```python
from build123d import *

# Parameters (mm, degrees)
CYLINDER005_R     = 2
CYLINDER005_DEPTH = 10
CYLINDER004_R     = 2
CYLINDER004_DEPTH = 10
CYLINDER003_R     = 2
CYLINDER003_DEPTH = 10
CYLINDER002_R     = 2
CYLINDER002_DEPTH = 10
CYLINDER001_R     = 2
CYLINDER001_DEPTH = 10
CYLINDER_R        = 2
CYLINDER_DEPTH    = 10
BOX_W             = 20
BOX_H             = 14
BOX_DEPTH         = 10


with BuildPart() as cilindro005:
    # Cylinder005 → Cylinder005 (new body)
    with BuildSketch(Plane(origin=(16, 10, 0), x_dir=(1, 0, 0), z_dir=(0, 0, 1))):
        Circle(CYLINDER005_R)
    extrude(amount=CYLINDER005_DEPTH)


with BuildPart() as cilindro004:
    # Cylinder004 → Cylinder004 (new body)
    with BuildSketch(Plane(origin=(16, 4, 0), x_dir=(1, 0, 0), z_dir=(0, 0, 1))):
        Circle(CYLINDER004_R)
    extrude(amount=CYLINDER004_DEPTH)


with BuildPart() as cilindro003:
    # Cylinder003 → Cylinder003 (new body)
    with BuildSketch(Plane(origin=(10, 10, 0), x_dir=(1, 0, 0), z_dir=(0, 0, 1))):
        Circle(CYLINDER003_R)
    extrude(amount=CYLINDER003_DEPTH)


with BuildPart() as cilindro002:
    # Cylinder002 → Cylinder002 (new body)
    with BuildSketch(Plane(origin=(10, 4, 0), x_dir=(1, 0, 0), z_dir=(0, 0, 1))):
        Circle(CYLINDER002_R)
    extrude(amount=CYLINDER002_DEPTH)


with BuildPart() as cilindro001:
    # Cylinder001 → Cylinder001 (new body)
    with BuildSketch(Plane(origin=(4, 10, 0), x_dir=(1, 0, 0), z_dir=(0, 0, 1))):
        Circle(CYLINDER001_R)
    extrude(amount=CYLINDER001_DEPTH)


with BuildPart() as cilindro:
    # Cylinder → Cylinder (new body)
    with BuildSketch(Plane(origin=(4, 4, 0), x_dir=(1, 0, 0), z_dir=(0, 0, 1))):
        Circle(CYLINDER_R)
    extrude(amount=CYLINDER_DEPTH)


with BuildPart() as cut005:
    # Box → Box (new body)
    with BuildSketch(Plane.XY):
        with Locations((10, 7)):
            Rectangle(BOX_W, BOX_H)
    extrude(amount=BOX_DEPTH)

    # Cut: cut Cilindro
    add(cilindro.part, mode=Mode.SUBTRACT)

    # Cut001: cut Cilindro001
    add(cilindro001.part, mode=Mode.SUBTRACT)

    # Cut002: cut Cilindro002
    add(cilindro002.part, mode=Mode.SUBTRACT)

    # Cut003: cut Cilindro003
    add(cilindro003.part, mode=Mode.SUBTRACT)

    # Cut004: cut Cilindro004
    add(cilindro004.part, mode=Mode.SUBTRACT)

    # Cut005: cut Cilindro005
    add(cilindro005.part, mode=Mode.SUBTRACT)


solid = cut005.part
```
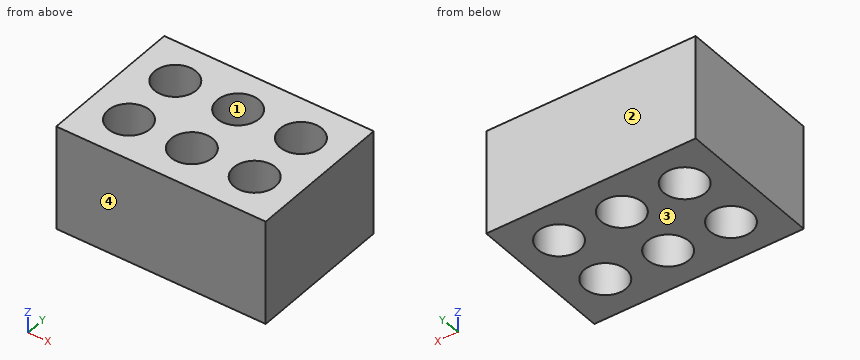
Geometry: final body of the model. Coordinates: model frame, mm. Face numbers are marked on the shaded views. Coordinates: 2 decimals unless noted, no trailing zeros. Loops run counter-clockwise (first coordinate to the right, second up) from the corner with the lowest first, then second, coordinate; pieces in that order, holes last. Notation, with made-up numbers: M 61,59.5 L 108,59.5 A12 cw 108,74.5 Z; hole C -28.75,-37.75 d8. An arc over 180 degrees is marked long. Put each result on its own line as item: value.
(1) Draft query along Y for the marked faces 1, 2, 3 and 4. Return one class per face: pulls with the +Y half, pulls with the -Y half, needs draft (parallel to the pull), parting line crosses it, or undercut.
Answer sheet:
face 1: undercut
face 2: pulls with the +Y half
face 3: needs draft
face 4: pulls with the -Y half
(2) Cut plane A-A on y = 4. Return the cut outline in (x, z), then the cut area to 3 significant figures.
Answer sheet:
outline: M 0,0 L 2,0 L 2,10 L 0,10 Z; M 6,0 L 8,0 L 8,10 L 6,10 Z; M 12,0 L 14,0 L 14,10 L 12,10 Z; M 18,0 L 20,0 L 20,10 L 18,10 Z
area: 80.0 mm^2
(3) Cut plane D-D on y = 8.25. Return the cut outline in (x, z).
Answer sheet:
outline: M 0,0 L 3.03,0 L 3.03,10 L 0,10 Z; M 4.97,0 L 9.03,0 L 9.03,10 L 4.97,10 Z; M 10.97,0 L 15.03,0 L 15.03,10 L 10.97,10 Z; M 16.97,0 L 20,0 L 20,10 L 16.97,10 Z
(4) Material intervals for probe 1 along Y at (x, z) = (16, 3.5); probe 2 along Y at (x, z) = (8.25, 0.75); probe 3 along X at (y, z) = (10.5, 6.5), sorted ascending.
Answer sheet:
probe 1: y = 0 to 2, 6 to 8, 12 to 14
probe 2: y = 0 to 3.03, 4.97 to 9.03, 10.97 to 14
probe 3: x = 0 to 2.06, 5.94 to 8.06, 11.94 to 14.06, 17.94 to 20
(5) Cut plane B-B on x = 4. Return the cut outline in (y, z).
Answer sheet:
outline: M 0,0 L 2,0 L 2,10 L 0,10 Z; M 6,0 L 8,0 L 8,10 L 6,10 Z; M 12,0 L 14,0 L 14,10 L 12,10 Z
(6) Cut plane C-C on z = 6.25. Return the cut outline in (x, y), then the cut area to 3 significant figures.
Answer sheet:
outline: M 0,0 L 20,0 L 20,14 L 0,14 Z; hole C 4,4 d4; hole C 4,10 d4; hole C 10,4 d4; hole C 10,10 d4; hole C 16,4 d4; hole C 16,10 d4
area: 205 mm^2
